The listing builds one solid part. Answer for the finished solid, in the listing's coordinates (mm). A direction names the side the tool comes from. Round coordinates to 2 decimals unless told otherwise and drop trailing zeros. Order: outer loops, then holes, each group sorted by start corner. A loop starts at its lowest first (then second) coordinate and runs counter-clockwise, first axis right, second up. Notation, with made-up numbers: (65, 24) - (91, 24) arc R25 ccw to (91, 55) - close; hole circle Ø7 at (-4.5, 68). An arc over 180 degrees is marked (long way). One line per item, written item: value. Start each with the question number.
1. Flat-ended cylindrical pins translate along their axes: P1, Ø3, axis at y = -10.5, z = -5, coming from the +X side; P2, Ø2, axis at x = 0.5, z = 2.5, coming from the +Y side; P3, Ø1.3, axis at x = 2.5, z = -6, coming from the -Y side. Find the tip coordinate at first contact, or state that the pin passes through.
2. Section A-A, the plane y = -42 is taken. Give the vertices of the cut face in (x, z), then the cut area to 3 significant figures.
3. For a pull along X with two mould halves and no side action, classify faces 1 (the flat face through (0, -55, -2.99)), 2 (the flat face through (-6.4, -50, 1)), 3 (the cylindrical face through (4.363, 4.843, -0.573)), 4 (the cylindrical face through (-3.89, 4.93, -5.08)) as released by +X, released by -X, zero draft, split by the parting line, or undercut.
4. Straight lines are drawn through the part: line 1 (X direction, y = 4, z = 0); line 2 (Z direction, x = 4.75, y = -42); line 3 (Y direction, x = -2, z = -4). For each, find the intervals that lie inside material, in ascending order.
5. A tool of negligible diameter and unlimited length cuts with its end or side. For faces 5 (the flat face through (0, 0, 0)), 6 (the flat face through (0, -30, -4)), 7 (the flat face through (0.09, -62.74, 1.64)), from which of +Z, -Z, +X, -X, +Y, -Y can it reach the whole face along a straight path? Write none if from no direction.
from build123d import *

# Parameters (mm, degrees)
SKETCH1_R                       = 6.4
SKETCH1_R_2                     = 4.4
BOSS_EXTRUDE1_DEPTH             = 10
CHAMFER1_SIZE                   = 1
CHAMFER1_SIZE2                  = 0.176326981
BOSS_EXTRUDE2_START             = -30
SKETCH4_W                       = 12.8
SKETCH4_H                       = 9.39
SKETCH4_H_2                     = 1.21
BOSS_EXTRUDE2_DEPTH             = 15
BOSS_EXTRUDE3_REACH             = 47.901
BOSS_EXTRUDE3_DIRECTION_2_REACH = 47.901


with BuildPart() as part:
    # Sketch1 → Boss-Extrude1 (new body)
    with BuildSketch(Plane(origin=(0, 0, 0), x_dir=(1, 0, 0), z_dir=(0, 1, 0))):
        with Locations(Location((0, 0, 0), (0, 0, 270))):
            Circle(SKETCH1_R)
        with Locations(Location((0, 0, 0), (0, 0, 270))):
            Circle(SKETCH1_R_2, mode=Mode.SUBTRACT)
    extrude(amount=BOSS_EXTRUDE1_DEPTH)

    # Chamfer1
    chamfer1_edges = [part.edges().sort_by_distance(p)[0] for p in [
        (0, 10, -4.4),
    ]]
    chamfer1_side = [part.faces().sort_by_distance(p)[0] for p in [
        (0, 10, -6.218980664),
    ]]
    chamfer(chamfer1_edges, length=CHAMFER1_SIZE, length2=CHAMFER1_SIZE2, reference=chamfer1_side[0])

    # Sketch2 for Loft1 → Loft1 section 0
    with BuildSketch(Plane.XZ):
        with BuildLine():
            # circular arc as an exact rational Bezier (weights 1, cos(half-angle), 1)
            Bezier((-4.5254834, -4.5254834), (0, -9.050966798), (4.5254834, -4.5254834), weights=[1, 0.707106781, 1])
            Bezier((4.5254834, -4.5254834), (9.050966798, 0), (4.5254834, 4.5254834), weights=[1, 0.707106781, 1])
            Bezier((4.5254834, 4.5254834), (0, 9.050966798), (-4.5254834, 4.5254834), weights=[1, 0.707106781, 1])
            Bezier((-4.5254834, 4.5254834), (-9.050966798, 0), (-4.5254834, -4.5254834), weights=[1, 0.707106781, 1])
        make_face()
    # Sketch3 → Loft1 section 1
    with BuildSketch(Plane(origin=(0, -30, 0), x_dir=(-1, 0, 0), z_dir=(0, -1, 0))):
        with BuildLine():
            Line((6.4, 6.4), (-6.4, 6.4))
            Line((-6.4, 6.4), (-6.4, -6.4))
            Line((-6.4, -6.4), (6.4, -6.4))
            Line((6.4, -6.4), (6.4, 6.4))
        make_face()
    loft()

    # Sketch4 → Boss-Extrude2 (add)
    with BuildSketch(Plane(origin=(0, 0, 0), x_dir=(1, 0, 0), z_dir=(0, 1, 0)).offset(BOSS_EXTRUDE2_START)):
        with Locations((0, -1.705)):
            Rectangle(SKETCH4_W, SKETCH4_H)
        with Locations((0, 5.795)):
            Rectangle(SKETCH4_W, SKETCH4_H_2)
    extrude(amount=-BOSS_EXTRUDE2_DEPTH)

    # Boss-Extrude3: up to this face of the body (flat: up to its plane)
    boss_extrude3_end = Plane(part.part.faces().sort_by_distance((6.4, -37.5, 1.705))[0])
    # Sketch5 → Boss-Extrude3 (add, up to the picked face)
    with BuildSketch(Plane(origin=(0, 0, 0), x_dir=(0, 0, -1), z_dir=(1, 0, 0)), mode=Mode.PRIVATE) as boss_extrude3_sk1:
        Polygon((2.99, -45), (2.99, -80), (-6.4, -45), align=None)
    boss_extrude3_tool1 = split(extrude(boss_extrude3_sk1.sketch, amount=BOSS_EXTRUDE3_REACH, mode=Mode.PRIVATE), bisect_by=boss_extrude3_end, keep=Keep.BOTH, mode=Mode.PRIVATE)
    add(boss_extrude3_tool1.solids().sort_by(Axis((0, -56.666667, 0.14), (1, 0, 0)))[0])

    # Boss-Extrude3 direction 2: up to this face of the body (flat: up to its plane)
    boss_extrude3_direction_2_end = Plane(part.part.faces().sort_by_distance((-6.4, -37.5, 1.705))[0])
    # Sketch5 → Boss-Extrude3 direction 2 (add, up to the picked face)
    with BuildSketch(Plane(origin=(0, 0, 0), x_dir=(0, 0, -1), z_dir=(1, 0, 0)), mode=Mode.PRIVATE) as boss_extrude3_direction_2_sk1:
        Polygon((2.99, -45), (2.99, -80), (-6.4, -45), align=None)
    boss_extrude3_direction_2_tool1 = split(extrude(boss_extrude3_direction_2_sk1.sketch, amount=-BOSS_EXTRUDE3_DIRECTION_2_REACH, mode=Mode.PRIVATE), bisect_by=boss_extrude3_direction_2_end, keep=Keep.BOTH, mode=Mode.PRIVATE)
    add(boss_extrude3_direction_2_tool1.solids().sort_by(Axis((0, -56.666667, 0.14), (-1, 0, 0)))[0])


solid = part.part
Answer list:
1. P1: stops at x = 5.86
1. P2: stops at y = 0
1. P3: stops at y = -45
2. outline: (-6.4, -6.4) - (6.4, -6.4) - (6.4, -5.19) - (-6.4, -5.19) - close; (-6.4, -2.99) - (6.4, -2.99) - (6.4, 6.4) - (-6.4, 6.4) - close
2. area: 136 mm²
3. face 1: zero draft
3. face 2: released by -X
3. face 3: undercut
3. face 4: split by the parting line
4. line 1: x = -6.4 to -4.4, 4.4 to 6.4
4. line 2: z = -6.4 to -5.19, -2.99 to 6.4
4. line 3: y = -30 to 9.84
5. face 5: +Y
5. face 6: +X, -X, -Y
5. face 7: +Z, +X, -X, -Y
